from build123d import *

# Parameters (mm, degrees)
SKETCH057_R     = 21
SKETCH057_R_2   = 12.5
PAD034_DEPTH    = 9
CHAMFER_SIZE    = 0.5
CHAMFER001_SIZE = 0.5


with BuildPart() as part:
    # Sketch057 → Pad034 (new body)
    with BuildSketch(Plane.XZ.offset(-122.5)):
        Circle(SKETCH057_R)
        Circle(SKETCH057_R_2, mode=Mode.SUBTRACT)
    extrude(amount=-PAD034_DEPTH)

    # Chamfer
    chamfer_edges = [part.edges().sort_by_distance(p)[0] for p in [
        (-21, 122.5, 0),
        (-12.5, 122.5, 0),
    ]]
    chamfer(chamfer_edges, length=CHAMFER_SIZE)

    # Chamfer001
    chamfer001_edges = [part.edges().sort_by_distance(p)[0] for p in [
        (-21, 131.5, 0),
        (-12.5, 131.5, 0),
    ]]
    chamfer(chamfer001_edges, length=CHAMFER001_SIZE)


solid = part.part
Can you work these out from the model? Positions are in its coordinate system, mm. Give positions to 0.01 mm unless a question says otherwise; leave off trailing zeros. Loops run counter-clockwise (first coordinate to the right, second up) from the corner with the lowest first, then second, coordinate; pieces in that order, holes last. Notation, with made-up numbers: (43.25, 76) -> (96.25, 76) arc R34 cw to (96.25, 115) -> close; hole circle Ø4 at (-5.5, 73.25). An arc over 180 degrees is marked (long way). Return JSON: item names as keys, results as strings.
Q1. I want a section at A-A, the plane z = 0. List the corners of the cut face in (x, y) for me.
Checks:
{"outline": "(-21, 123) -> (-20.5, 122.5) -> (-13, 122.5) -> (-12.5, 123) -> (-12.5, 131) -> (-13, 131.5) -> (-20.5, 131.5) -> (-21, 131) -> close; (12.5, 123) -> (13, 122.5) -> (20.5, 122.5) -> (21, 123) -> (21, 131) -> (20.5, 131.5) -> (13, 131.5) -> (12.5, 131) -> close"}
Q2. I want a section at C-C, the plane y = 126.75. List the corners of the cut face in (x, z) for me.
Checks:
{"outline": "circle Ø42 at (0, 0); hole circle Ø25 at (0, 0)"}
Q3. For pin 1 Ø1 at (x, y) = (5.5, 128) entering from +Z; pin 2 Ø1 at (y, z) = (129.5, -3) entering from +X; pin 3 Ø4 at (x, y) = (2, 126) entering from -Z; pin 4 Ø8 at (x, z) = (-2, 10.5) entering from -Y, each with a flat end and sliding along its axis, tell me the tip position at first contact or that it passes through.
Checks:
{"pin 1": "stops at z = 20.4", "pin 2": "stops at x = 20.85", "pin 3": "stops at z = -21", "pin 4": "stops at y = 122.5"}
Q4. I want a section at B-B, the plane x = 0. List the corners of the cut face in (y, z) for me, then the cut area to 3 significant figures.
Checks:
{"outline": "(122.5, -20.5) -> (123, -21) -> (131, -21) -> (131.5, -20.5) -> (131.5, -13) -> (131, -12.5) -> (123, -12.5) -> (122.5, -13) -> close; (122.5, 13) -> (123, 12.5) -> (131, 12.5) -> (131.5, 13) -> (131.5, 20.5) -> (131, 21) -> (123, 21) -> (122.5, 20.5) -> close", "area": "152 mm2"}
Q5. We'd pull the mould along X, two halves only. Please class faces 1 (the face through (20.03, 126.94, 6.31)), 2 (the face through (13.4, 131.5, 0.3)), 3 (the face through (11.923, 126.944, 3.755)): released by +X, released by -X, zero draft, split by the parting line, or undercut.
Checks:
{"face 1": "split by the parting line", "face 2": "zero draft", "face 3": "undercut"}
Q6. I need wall thicknesses on probe 1 along Z at (x, y) = (0, 127.5); probe 2 along Z at (x, y) = (9, 126); probe 3 along X at (y, z) = (127.75, 11.5). Which ranges of each line are inside material? Lowest first, please.
Checks:
{"probe 1": "z = -21 to -12.5, 12.5 to 21", "probe 2": "z = -18.97 to -8.67, 8.67 to 18.97", "probe 3": "x = -17.57 to -4.9, 4.9 to 17.57"}
